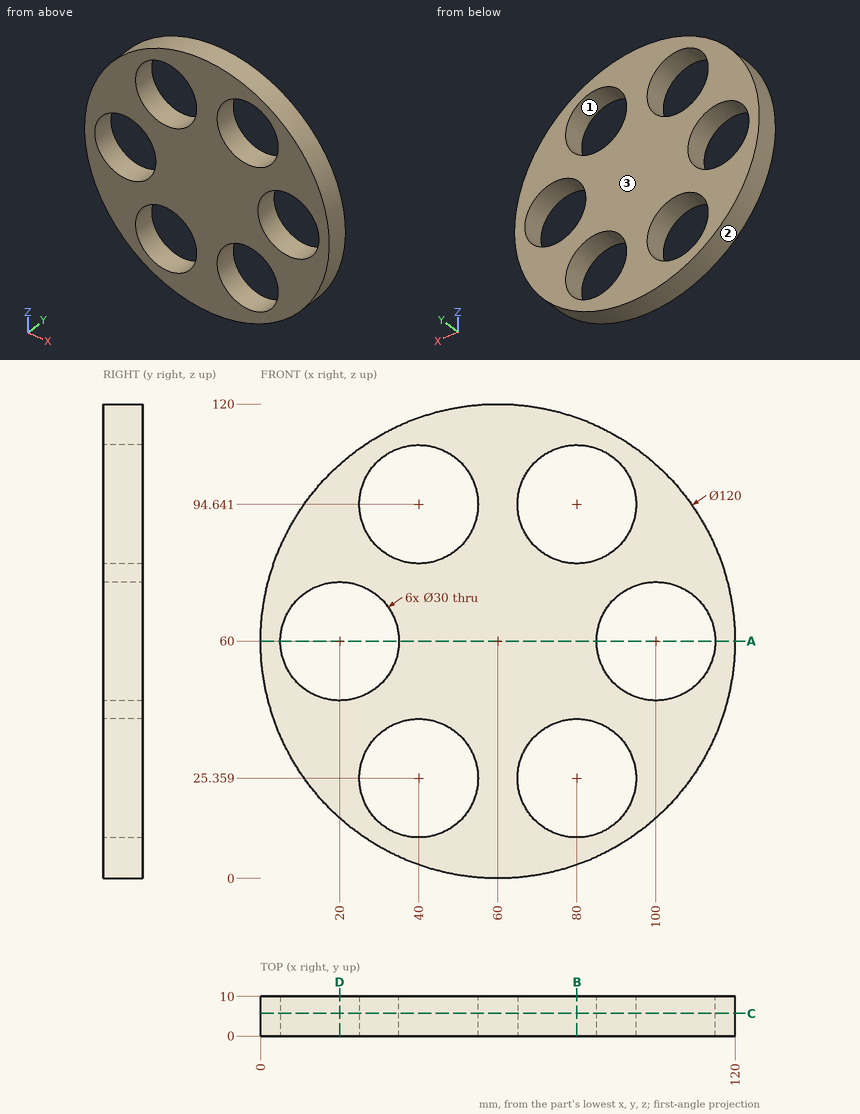
Here's the drawing with two shaded views (mm, measured from the low corner). I have some questions. Coordinates: 2 decimals unless noted, no trailing zeros. Write each loop counter-clockwise with the first axis right and the second up, starting at its lowest first coordinate (ties: lowest second). Pieces come first, ordered by that corner, then holes.
Item 1: I want a section at C-C on y = 5.75. Write out the boundary of the cut face in (x, z), and give its area (3 significant figures).
Item 2: If we mould it in two halves opening along Z, with no side actions, what happens to the marked faces 1, 2 and 3? For each: +Z half, -Z half, draft (parallel to the pull), parting line (faces both ways), or undercut.
Item 3: I want a section at A-A on z = 60. Write out the boundary of the cut face in (x, y).
Item 4: I want a section at B-B on x = 80. Write out the boundary of the cut face in (y, z), and give its area (3 significant figures).
Item 5: If I drill on line 1 (Z direction, x = 80, y = 7.25); line 2 (Z direction, x = 27, y = 9); line 3 (X direction, y = 9, z = 97.5) (1 decimal), over which ranges is the centre line in solid material (lowest first)?
Item 6: I want a section at D-D on x = 20. Write out the boundary of the cut face in (y, z).
Item 7: Will these pins go through, and if not, where does the flat tip stop? pin 1 (1.5 mm diameter, centred on y = 7, z = 105, fed in from +X); pin 2 (18 mm diameter, centred on x = 80, z = 94.64, fed in from -Y); pin 3 (5 mm diameter, centred on x = 97, y = 5.5, fed in from +Z); pin 4 (4 mm diameter, centred on x = 72, y = 5.5, fed in from +Z).
Findings below:
1. outline: circle Ø120 at (60, 60); hole circle Ø30 at (20, 60); hole circle Ø30 at (40, 25.36); hole circle Ø30 at (40, 94.64); hole circle Ø30 at (80, 25.36); hole circle Ø30 at (80, 94.64); hole circle Ø30 at (100, 60)
1. area: 7,070 mm2
2. face 1: undercut
2. face 2: parting line
2. face 3: draft
3. outline: (0, 0) - (5, 0) - (5, 10) - (0, 10) - close; (35, 0) - (85, 0) - (85, 10) - (35, 10) - close; (115, 0) - (120, 0) - (120, 10) - (115, 10) - close
4. outline: (0, 3.43) - (10, 3.43) - (10, 10.36) - (0, 10.36) - close; (0, 40.36) - (10, 40.36) - (10, 79.64) - (0, 79.64) - close; (0, 109.64) - (10, 109.64) - (10, 116.57) - (0, 116.57) - close
4. area: 531 mm2
5. line 1: z = 3.43 to 10.36, 40.36 to 79.64, 109.64 to 116.57
5. line 2: z = 9.89 to 17.88, 32.84 to 46.73, 73.27 to 87.16, 102.12 to 110.11
5. line 3: x = 13.2 to 25.3, 54.7 to 65.3, 94.7 to 106.8
6. outline: (0, 15.28) - (10, 15.28) - (10, 45) - (0, 45) - close; (0, 75) - (10, 75) - (10, 104.72) - (0, 104.72) - close
7. pin 1: stops at x = 100.52
7. pin 2: passes through
7. pin 3: stops at z = 109.09
7. pin 4: stops at z = 119.16
